Part model, mm, in its own coordinate system. Coordinates: 2 decimals unless noted, no trailing zeros. Order: outer loops, then holes, each group sorted by start corner. A loop starts at its lowest first (then second) coordinate and runs counter-clockwise, first axis right, second up. Notation, with made-up numbers: M -4,2 L 21,2 A15 ccw 21,8 Z; hole C 45,74 d6. An arc over 180 degrees is marked long. Write item = value, one per line. Start each with the question number.
from build123d import *

# Parameters (mm, degrees)
F0_W         = 120.65
F0_H         = 22.225
F0_W_2       = 107.95
F0_H_2       = 9.525
F1_DEPTH     = 165.1
F2_W         = 22.225
F2_H         = 6.35
F3_DEPTH     = 55.88
F5_T1_DEPTH  = 113.03
F5_T3_DEPTH  = 27.94
F5_T5_DEPTH  = 157.48
F5_T7_DEPTH  = 9.525
F5_T9_DEPTH  = 107.95
F5_S13_W     = 3.81
F5_S13_H     = 3.81
F5_T14_DEPTH = 3.81
F5_S19_W     = 3.81
F5_S19_H     = 3.81
F5_T20_DEPTH = 3.81
F5_S25_W     = 3.81
F5_S25_H     = 3.81
F5_T26_DEPTH = 3.81
F5_S31_W     = 3.81
F5_S31_H     = 3.81
F5_T32_DEPTH = 3.81
F5_T39_DEPTH = 117.475
F5_T43_DEPTH = 19.05
F5_T50_DEPTH = 19.05
F5_T54_DEPTH = 117.475
F5_T61_DEPTH = 19.05
F5_T65_DEPTH = 117.475
F5_T72_DEPTH = 19.05
F5_T76_DEPTH = 117.475
F4_W         = 13.208
F4_H         = 144.78
F6_DEPTH     = 40.64


# Not quite as in the source:
# - a fillet or chamfer that OpenCascade refuses, or shapes differently, is made with other operations: its cross-section is extruded or revolved along the edge and cut away or added
# - a feature names something its author has since deleted; it is built from what else it names


with BuildPart() as f1:
    # F0 (on Top) → F1 (new body)
    with BuildSketch(Plane.XY):
        Rectangle(F0_W, F0_H)
        Rectangle(F0_W_2, F0_H_2, mode=Mode.SUBTRACT)
    extrude(amount=F1_DEPTH)

    # F2 (on Right) → F3 (join, symmetric)
    with BuildSketch(Plane.YZ):
        with Locations((0, 3.175)):
            Rectangle(F2_W, F2_H)
    extrude(amount=F3_DEPTH, both=True)

    # F5: fillet of radius 3.81 on 12 edges, made by hand

    # F5_s2 → F5_t1 (cut)
    with BuildSketch(Plane.YZ.offset(-56.515)):
        with BuildLine():
            ThreePointArc((-11.1125, 161.29), (-9.9965768363, 163.9840768363), (-7.3025, 165.1))
            Line((-7.3025, 165.1), (-11.1125, 165.1))
            Line((-11.1125, 165.1), (-11.1125, 161.29))
        make_face()
        with BuildLine():
            ThreePointArc((-11.1125, 3.81), (-9.9965768363, 1.1159231637), (-7.3025, 0))
            Line((-7.3025, 0), (-11.1125, 0))
            Line((-11.1125, 0), (-11.1125, 3.81))
        make_face()
    extrude(amount=F5_T1_DEPTH, mode=Mode.SUBTRACT)

    # F5_s4 → F5_t3 (cut)
    with BuildSketch(Plane.XZ.offset(-20.6375)):
        with BuildLine():
            ThreePointArc((-60.325, 161.29), (-59.2090768363, 163.9840768363), (-56.515, 165.1))
            Line((-56.515, 165.1), (-60.325, 165.1))
            Line((-60.325, 165.1), (-60.325, 161.29))
        make_face()
        with BuildLine():
            ThreePointArc((56.515, 165.1), (59.2090768363, 163.9840768363), (60.325, 161.29))
            Line((60.325, 161.29), (60.325, 165.1))
            Line((60.325, 165.1), (56.515, 165.1))
        make_face()
        with BuildLine():
            ThreePointArc((60.325, 3.81), (59.2090768363, 1.1159231637), (56.515, 0))
            Line((56.515, 0), (60.325, 0))
            Line((60.325, 0), (60.325, 3.81))
        make_face()
        with BuildLine():
            ThreePointArc((-60.325, 3.81), (-59.2090768363, 1.1159231637), (-56.515, 0))
            Line((-56.515, 0), (-60.325, 0))
            Line((-60.325, 0), (-60.325, 3.81))
        make_face()
    extrude(amount=F5_T3_DEPTH, mode=Mode.SUBTRACT)

    # F5_s6 → F5_t5 (cut)
    with BuildSketch(Plane.XY.offset(3.81)):
        with BuildLine():
            ThreePointArc((56.515, -11.1125), (59.2090768363, -9.9965768363), (60.325, -7.3025))
            Line((60.325, -7.3025), (60.325, -11.1125))
            Line((60.325, -11.1125), (56.515, -11.1125))
        make_face()
        with BuildLine():
            ThreePointArc((-60.325, -7.3025), (-59.2090768363, -9.9965768363), (-56.515, -11.1125))
            Line((-56.515, -11.1125), (-60.325, -11.1125))
            Line((-60.325, -11.1125), (-60.325, -7.3025))
        make_face()
    extrude(amount=F5_T5_DEPTH, mode=Mode.SUBTRACT)

    # F5_s8 → F5_t7 (cut)
    with BuildSketch(Plane.XZ.offset(-4.7625)):
        with BuildLine():
            ThreePointArc((57.785, 165.1), (55.0909231637, 163.9840768363), (53.975, 161.29))
            Line((53.975, 161.29), (53.975, 165.1))
            Line((53.975, 165.1), (57.785, 165.1))
        make_face()
        with BuildLine():
            ThreePointArc((-57.785, 165.1), (-55.0909231637, 163.9840768363), (-53.975, 161.29))
            Line((-53.975, 161.29), (-53.975, 165.1))
            Line((-53.975, 165.1), (-57.785, 165.1))
        make_face()
    extrude(amount=F5_T7_DEPTH, mode=Mode.SUBTRACT)

    # F5_s10 → F5_t9 (cut)
    with BuildSketch(Plane.YZ.offset(-53.975)):
        with BuildLine():
            ThreePointArc((-8.5725, 165.1), (-5.8784231637, 163.9840768363), (-4.7625, 161.29))
            Line((-4.7625, 161.29), (-4.7625, 165.1))
            Line((-4.7625, 165.1), (-8.5725, 165.1))
        make_face()
        with BuildLine():
            ThreePointArc((8.5725, 165.1), (5.8784231637, 163.9840768363), (4.7625, 161.29))
            Line((4.7625, 161.29), (4.7625, 165.1))
            Line((4.7625, 165.1), (8.5725, 165.1))
        make_face()
    extrude(amount=F5_T9_DEPTH, mode=Mode.SUBTRACT)


with BuildPart() as f5_tool12:
    # F5_s13 → F5_t14 (new body)
    with BuildSketch(Plane.YZ.offset(-56.515)):
        with Locations((-9.2075, 163.195)):
            Rectangle(F5_S13_W, F5_S13_H)
    extrude(amount=-F5_T14_DEPTH)

    # F5_s15 → F5_t16 (revolve, cut)
    with BuildSketch(Plane(origin=(-56.515, -7.3025, 161.29), x_dir=(0, 0.7071067812, -0.7071067812), z_dir=(0, 0.7071067812, 0.7071067812))):
        with BuildLine():
            ThreePointArc((0, -3.81), (3.81, 0), (0, 3.81))
            Line((0, 3.81), (0, -3.81))
        make_face()
    revolve(axis=Axis((-56.515, -7.3025, 161.29), (-1, 0, 0)), mode=Mode.SUBTRACT)


with BuildPart() as f1_1:
    add(f1.part)

    # F5_t11: cut F5_tool12
    add(f5_tool12.part, mode=Mode.SUBTRACT)


with BuildPart() as f5_tool18:
    # F5_s19 → F5_t20 (new body)
    with BuildSketch(Plane.YZ.offset(56.515)):
        with Locations((-9.2075, 163.195)):
            Rectangle(F5_S19_W, F5_S19_H)
    extrude(amount=F5_T20_DEPTH)

    # F5_s21 → F5_t22 (revolve, cut)
    with BuildSketch(Plane(origin=(56.515, -7.3025, 161.29), x_dir=(0, 0.7071067812, -0.7071067812), z_dir=(0, -0.7071067812, -0.7071067812))):
        with BuildLine():
            ThreePointArc((0, -3.81), (3.81, 0), (0, 3.81))
            Line((0, 3.81), (0, -3.81))
        make_face()
    revolve(axis=Axis((56.515, -7.3025, 161.29), (1, 0, 0)), mode=Mode.SUBTRACT)


with BuildPart() as f1_2:
    add(f1_1.part)

    # F5_t17: cut F5_tool18
    add(f5_tool18.part, mode=Mode.SUBTRACT)


with BuildPart() as f5_tool24:
    # F5_s25 → F5_t26 (new body)
    with BuildSketch(Plane.YZ.offset(56.515)):
        with Locations((-9.2075, 1.905)):
            Rectangle(F5_S25_W, F5_S25_H)
    extrude(amount=F5_T26_DEPTH)

    # F5_s27 → F5_t28 (revolve, cut)
    with BuildSketch(Plane(origin=(56.515, -7.3025, 3.81), x_dir=(0, 0.7071067812, 0.7071067812), z_dir=(0, 0.7071067812, -0.7071067812))):
        with BuildLine():
            ThreePointArc((0, -3.81), (3.81, 0), (0, 3.81))
            Line((0, 3.81), (0, -3.81))
        make_face()
    revolve(axis=Axis((56.515, -7.3025, 3.81), (1, 0, 0)), mode=Mode.SUBTRACT)


with BuildPart() as f1_3:
    add(f1_2.part)

    # F5_t23: cut F5_tool24
    add(f5_tool24.part, mode=Mode.SUBTRACT)


with BuildPart() as f5_tool30:
    # F5_s31 → F5_t32 (new body)
    with BuildSketch(Plane.YZ.offset(-56.515)):
        with Locations((-9.2075, 1.905)):
            Rectangle(F5_S31_W, F5_S31_H)
    extrude(amount=-F5_T32_DEPTH)

    # F5_s33 → F5_t34 (revolve, cut)
    with BuildSketch(Plane(origin=(-56.515, -7.3025, 3.81), x_dir=(0, 0.7071067812, 0.7071067812), z_dir=(0, -0.7071067812, 0.7071067812))):
        with BuildLine():
            ThreePointArc((0, -3.81), (3.81, 0), (0, 3.81))
            Line((0, 3.81), (0, -3.81))
        make_face()
    revolve(axis=Axis((-56.515, -7.3025, 3.81), (-1, 0, 0)), mode=Mode.SUBTRACT)


with BuildPart() as f1_4:
    add(f1_3.part)

    # F5_t29: cut F5_tool30
    add(f5_tool30.part, mode=Mode.SUBTRACT)


with BuildPart() as f5_tool37:
    # F5_s38 → F5_t39 (new body)
    with BuildSketch(Plane.YZ.offset(-53.975)):
        with BuildLine():
            ThreePointArc((8.5725, 165.1), (5.8784231637, 163.9840768363), (4.7625, 161.29))
            Line((4.7625, 161.29), (4.7625, 165.1))
            Line((4.7625, 165.1), (8.5725, 165.1))
        make_face()
    extrude(amount=F5_T39_DEPTH)

    split(bisect_by=Plane.YZ.offset(53.975), keep=Keep.TOP)


with BuildPart() as f5_tool41:
    # F5_s42 → F5_t43 (new body)
    with BuildSketch(Plane.XZ.offset(-14.2875)):
        with BuildLine():
            ThreePointArc((57.785, 165.1), (55.0909231637, 163.9840768363), (53.975, 161.29))
            Line((53.975, 161.29), (53.975, 165.1))
            Line((53.975, 165.1), (57.785, 165.1))
        make_face()
    extrude(amount=F5_T43_DEPTH)

    split(bisect_by=Plane.XZ.offset(-4.7625), keep=Keep.BOTTOM)


with BuildPart() as f5_tool37_1:
    add(f5_tool37.part)

    # F5_t45: intersect F5_tool41
    add(f5_tool41.part, mode=Mode.INTERSECT)


with BuildPart() as f1_5:
    add(f1_4.part)

    # F5_t35: cut F5_tool37
    add(f5_tool37_1.part, mode=Mode.SUBTRACT)


with BuildPart() as f5_tool48:
    # F5_s49 → F5_t50 (new body)
    with BuildSketch(Plane.XZ.offset(-4.7625)):
        with BuildLine():
            ThreePointArc((57.785, 165.1), (55.0909231637, 163.9840768363), (53.975, 161.29))
            Line((53.975, 161.29), (53.975, 165.1))
            Line((53.975, 165.1), (57.785, 165.1))
        make_face()
    extrude(amount=F5_T50_DEPTH)

    split(bisect_by=Plane.XZ.offset(4.7625), keep=Keep.TOP)


with BuildPart() as f5_tool52:
    # F5_s53 → F5_t54 (new body)
    with BuildSketch(Plane.YZ.offset(63.5)):
        with BuildLine():
            ThreePointArc((-8.5725, 165.1), (-5.8784231637, 163.9840768363), (-4.7625, 161.29))
            Line((-4.7625, 161.29), (-4.7625, 165.1))
            Line((-4.7625, 165.1), (-8.5725, 165.1))
        make_face()
    extrude(amount=-F5_T54_DEPTH)

    split(bisect_by=Plane.YZ.offset(53.975), keep=Keep.TOP)


with BuildPart() as f5_tool48_1:
    add(f5_tool48.part)

    # F5_t56: intersect F5_tool52
    add(f5_tool52.part, mode=Mode.INTERSECT)


with BuildPart() as f1_6:
    add(f1_5.part)

    # F5_t46: cut F5_tool48
    add(f5_tool48_1.part, mode=Mode.SUBTRACT)


with BuildPart() as f5_tool59:
    # F5_s60 → F5_t61 (new body)
    with BuildSketch(Plane.XZ.offset(14.2875)):
        with BuildLine():
            ThreePointArc((-57.785, 165.1), (-55.0909231637, 163.9840768363), (-53.975, 161.29))
            Line((-53.975, 161.29), (-53.975, 165.1))
            Line((-53.975, 165.1), (-57.785, 165.1))
        make_face()
    extrude(amount=-F5_T61_DEPTH)

    split(bisect_by=Plane.XZ.offset(4.7625), keep=Keep.TOP)


with BuildPart() as f5_tool63:
    # F5_s64 → F5_t65 (new body)
    with BuildSketch(Plane.YZ.offset(53.975)):
        with BuildLine():
            ThreePointArc((-8.5725, 165.1), (-5.8784231637, 163.9840768363), (-4.7625, 161.29))
            Line((-4.7625, 161.29), (-4.7625, 165.1))
            Line((-4.7625, 165.1), (-8.5725, 165.1))
        make_face()
    extrude(amount=-F5_T65_DEPTH)

    split(bisect_by=Plane.YZ.offset(-53.975), keep=Keep.BOTTOM)


with BuildPart() as f5_tool59_1:
    add(f5_tool59.part)

    # F5_t67: intersect F5_tool63
    add(f5_tool63.part, mode=Mode.INTERSECT)


with BuildPart() as f1_7:
    add(f1_6.part)

    # F5_t57: cut F5_tool59
    add(f5_tool59_1.part, mode=Mode.SUBTRACT)


with BuildPart() as f5_tool70:
    # F5_s71 → F5_t72 (new body)
    with BuildSketch(Plane.XZ.offset(4.7625)):
        with BuildLine():
            ThreePointArc((-57.785, 165.1), (-55.0909231637, 163.9840768363), (-53.975, 161.29))
            Line((-53.975, 161.29), (-53.975, 165.1))
            Line((-53.975, 165.1), (-57.785, 165.1))
        make_face()
    extrude(amount=-F5_T72_DEPTH)

    split(bisect_by=Plane.XZ.offset(-4.7625), keep=Keep.BOTTOM)


with BuildPart() as f5_tool74:
    # F5_s75 → F5_t76 (new body)
    with BuildSketch(Plane.YZ.offset(-63.5)):
        with BuildLine():
            ThreePointArc((8.5725, 165.1), (5.8784231637, 163.9840768363), (4.7625, 161.29))
            Line((4.7625, 161.29), (4.7625, 165.1))
            Line((4.7625, 165.1), (8.5725, 165.1))
        make_face()
    extrude(amount=F5_T76_DEPTH)

    split(bisect_by=Plane.YZ.offset(-53.975), keep=Keep.BOTTOM)


with BuildPart() as f5_tool70_1:
    add(f5_tool70.part)

    # F5_t78: intersect F5_tool74
    add(f5_tool74.part, mode=Mode.INTERSECT)


with BuildPart() as f1_8:
    add(f1_7.part)

    # F5_t68: cut F5_tool70
    add(f5_tool70_1.part, mode=Mode.SUBTRACT)

    # F4 (on face) → F6 (cut)
    with BuildSketch(Plane.XZ.offset(11.1125)):
        with Locations((-44.831, 83.82)):
            Rectangle(F4_W, F4_H)
        with Locations((-23.0886, 83.82)):
            Rectangle(F4_W, F4_H)
        with Locations((-1.3462, 83.82)):
            Rectangle(F4_W, F4_H)
        with Locations((20.3962, 83.82)):
            Rectangle(F4_W, F4_H)
        with Locations((42.1386, 83.82)):
            Rectangle(F4_W, F4_H)
    extrude(amount=-F6_DEPTH, mode=Mode.SUBTRACT)


solid = f1_8.part
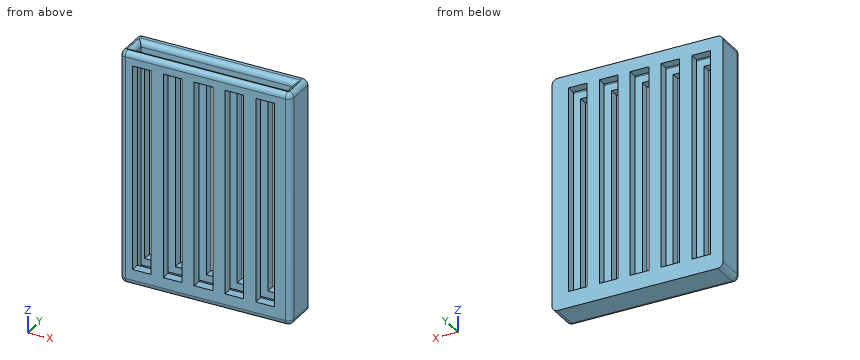
Item 1: Wall check: line 1 along X through (y, z) = (10, 50.5) (3 decimals); line 2 along X through (y, z) = (-3.25, 21.5) (3 decimals); line 3 along Y through (x, z) = (35, 68). Give the ranges that are in metal, low to high. Write a range as [from, to].
Item 2: Flat gauge pins, fed straight in: pin 1 (1 mm diameter, centred on y = -8.5, z = 24, fed in from +X); pin 2 (10 mm diameter, centred on x = -19.5, y = -7.5, fed in from +Z); pin 3 (10.5 mm diameter, centred on x = -22, y = 2, fed in from +Z). Where does each tip first touch, or does it go through?
Item 3: Cut at C-C, the plane y = -0.5. Write the cut outline in (x, z) (3 decimals), and give its area (3 significant figures).
Item 4: Cut at A-A, the plane z = 22.5. Count the separate pieces of the cut face and the enclosed holes in it, and give its area (3 significant figures).
Item 5: Cut at B-B, the plane x = -31.5. Write the cut outline in (y, z).
Filled sheet:
q1.line_1 = [-60.325, -51.435], [-38.227, -29.693], [-16.485, -7.95], [5.258, 13.792], [27, 35.535], [48.743, 60.325]
q1.line_2 = [-60.325, -53.975], [53.975, 60.325]
q1.line_3 = [-11.11, -4.76], [4.76, 11.11]
q2.pin_1 = 60.26
q2.pin_2 = 165.05
q2.pin_3 = 164.86
q3.outline = M -60.325,3.81 A3.81 ccw -56.515,0 L 56.515,0 A3.81 ccw 60.325,3.81 L 60.325,161.29 A3.81 ccw 57.15,165.047 A3.81 ccw 53.975,161.29 L 53.975,6.35 L -53.975,6.35 L -53.975,161.29 A3.81 ccw -57.15,165.047 A3.81 ccw -60.325,161.29 Z
q3.area = 2,760 mm2
q4.separate_pieces = 10
q4.enclosed_holes = 0
q4.area = 808 mm2
q5.outline = M -11.11,3.81 A3.81 ccw -7.3,0 L 11.11,0 L 11.11,165.1 L 8.57,165.1 A3.81 ccw 4.76,161.29 L 4.76,6.35 L -4.76,6.35 L -4.76,161.29 A3.81 ccw -7.94,165.05 A3.81 ccw -11.11,161.29 Z
